The model under review builds one solid part; all positions refer to its coordinate system, in mm. Coordinates: 2 decimals unless noted, no trailing zeros. Order: outer loops, then holes, each group sorted by start corner. A loop starts at its lowest first (then second) coordinate and runs counter-clockwise, first axis right, second up. Notation, with made-up numbers: (87.5, 55) - (119.5, 55) arc R16 cw to (119.5, 85) - close; hole circle Ø9 at (-30, -28.75). An arc over 180 degrees is marked (long way). Answer in a Markdown table with one row per item.
```python
from build123d import *

# Parameters (mm, degrees)
F0_W     = 22
F0_H     = 28
F0_R     = 1.3
F1_DEPTH = 1.778
F2_R     = 2.231507
F3_DEPTH = 0.889


with BuildPart() as f1:
    # F0 (on Top) → F1 (new body)
    with BuildSketch(Plane.XY):
        with Locations((0, 6.5)):
            Rectangle(F0_W, F0_H)
        with Locations((-9, -5.5)):
            Circle(F0_R, mode=Mode.SUBTRACT)
        with Locations((-9, 5.5)):
            Circle(F0_R, mode=Mode.SUBTRACT)
        with Locations((9, -5.5)):
            Circle(F0_R, mode=Mode.SUBTRACT)
        with Locations((9, 5.5)):
            Circle(F0_R, mode=Mode.SUBTRACT)
    extrude(amount=F1_DEPTH)

    # F2 (on face) → F3 (join)
    with BuildSketch(Plane.XY.offset(1.778)):
        Circle(F2_R)
    extrude(amount=F3_DEPTH)


solid = f1.part
```
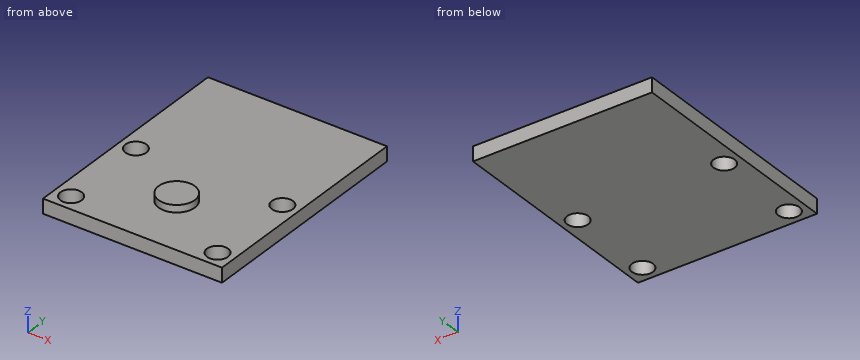
Item 1: We need section D-D, the plane x = 0. Write out the cut boundary in (y, z), then the cut area to 3 significant figures.
Check values:
| item | result |
|---|---|
| outline | (-7.5, 0) - (20.5, 0) - (20.5, 1.78) - (2.23, 1.78) - (2.23, 2.67) - (-2.23, 2.67) - (-2.23, 1.78) - (-7.5, 1.78) - close |
| area | 53.8 mm^2 |
Item 2: To check wall thickness, follow line 1 (Y direction, x = -9, z = 1.35); line 2 (Y direction, x = 10, z = 0.9); line 3 (Z direction, x = -7.75, y = 1.5). State the ranges of each line that lie inside material, in increasing order. Write a range as from..to.
Check values:
| item | result |
|---|---|
| line 1 | -7.5..-6.8, -4.2..4.2, 6.8..20.5 |
| line 2 | -7.5..-6.33, -4.67..4.67, 6.33..20.5 |
| line 3 | 0..1.78 |
Item 3: We need section C-C, the plane z = 1.2. Write out the cut boundary in (x, y), then the cut area to 3 significant figures.
Check values:
| item | result |
|---|---|
| outline | (-11, -7.5) - (11, -7.5) - (11, 20.5) - (-11, 20.5) - close; hole circle Ø2.6 at (-9, -5.5); hole circle Ø2.6 at (-9, 5.5); hole circle Ø2.6 at (9, -5.5); hole circle Ø2.6 at (9, 5.5) |
| area | 595 mm^2 |
Item 4: Clearance check with a flat-ended pin moving along its axis: pin 1 Ø5 at (x, y) = (4.5, 9) entering from +Z. State where the tip first meets the part, or that it passes through.
Check values:
| item | result |
|---|---|
| pin 1 | z = 1.78 |
Item 5: We need section B-B, the plane y = 5.5. Write out the cut boundary in (x, z), then the cut area to 3 significant figures.
Check values:
| item | result |
|---|---|
| outline | (-11, 0) - (-10.3, 0) - (-10.3, 1.78) - (-11, 1.78) - close; (-7.7, 0) - (7.7, 0) - (7.7, 1.78) - (-7.7, 1.78) - close; (10.3, 0) - (11, 0) - (11, 1.78) - (10.3, 1.78) - close |
| area | 29.9 mm^2 |
Item 6: We need section A-A, the plane x = -9. Write out the cut boundary in (y, z).
Check values:
| item | result |
|---|---|
| outline | (-7.5, 0) - (-6.8, 0) - (-6.8, 1.78) - (-7.5, 1.78) - close; (-4.2, 0) - (4.2, 0) - (4.2, 1.78) - (-4.2, 1.78) - close; (6.8, 0) - (20.5, 0) - (20.5, 1.78) - (6.8, 1.78) - close |
